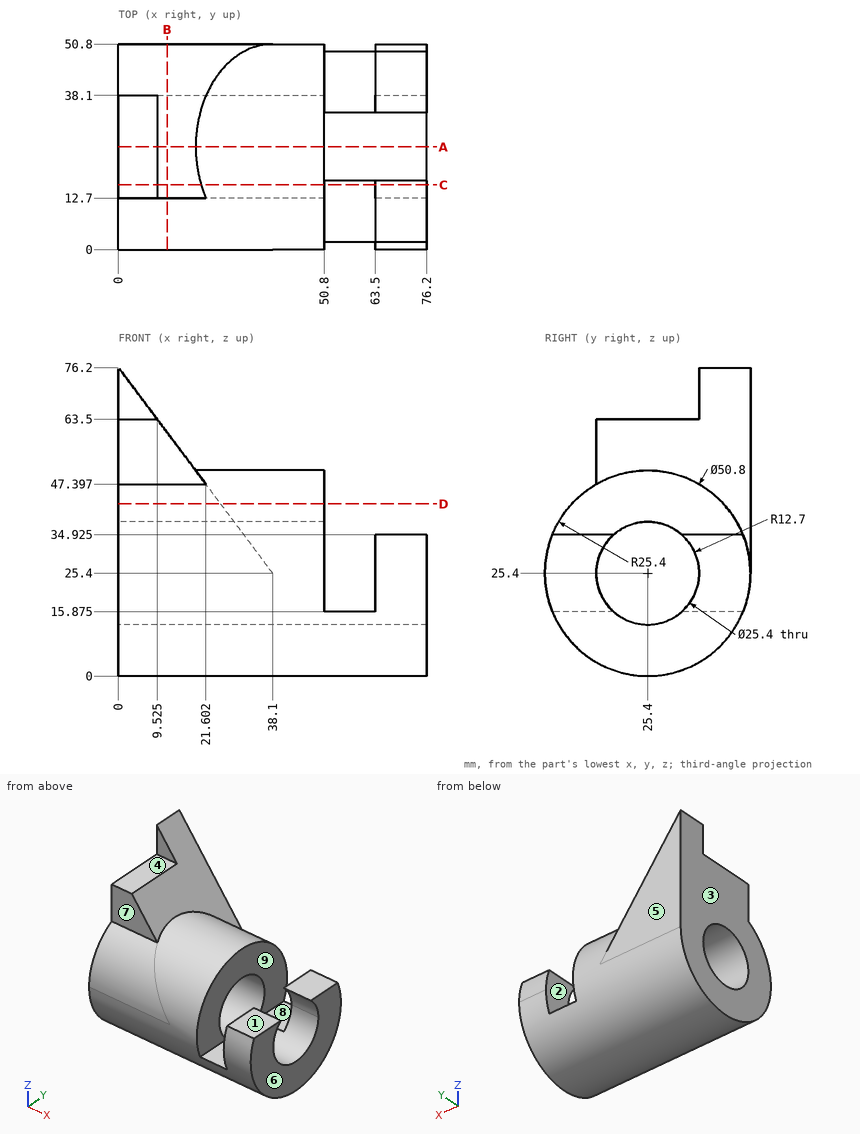
Answer from the drawing. Dimensions are ordinates in mm from the lowest x, y and z of the part. A direction names the side the tool comes from. Coordinates: 2 decimals unless noted, no trailing zeros. Order: outer loops, then holes, each group sorted by start corner. A loop starts at its lowest first (then second) coordinate and runs counter-clockwise, first axis right, second up. Notation, with made-up numbers: (-5.75, 55) - (6.25, 55) arc R21 ccw to (6.25, 82) - close; hole circle Ø2 at (11, 87.25). An arc over 180 degrees is marked (long way). Use one line per item in the form item = value.
(1) Section D-D, the plane z = 42.5 is taken. Give the vertices of the cut face in (x, y) (1 decimal).
Computed values:
outline = (0, 6.6) - (50.8, 6.6) - (50.8, 44.2) - (25.3, 44.2) - (25.3, 50.8) - (0, 50.8) - close
(2) For a pull along X with two mould halves and no side action, classify the marked faces 6, 7, 8 and 9 as pulls with the +X half, pulls with the -X half, needs draft (parallel to the pull), parting line crosses it, or undercut.
Computed values:
face_6 = pulls with the +X half
face_7 = needs draft
face_8 = undercut
face_9 = undercut
(3) Section C-C, the plane y = 16 is taken. Give the vertices of the cut face in (x, z) (1 decimal).
Computed values:
outline = (0, 1.8) - (76.2, 1.8) - (76.2, 16.9) - (63.5, 16.9) - (63.5, 15.9) - (50.8, 15.9) - (50.8, 16.9) - (0, 16.9) - close; (0, 33.9) - (50.8, 33.9) - (50.8, 49) - (20.4, 49) - (9.5, 63.5) - (0, 63.5) - close; (63.5, 33.9) - (76.2, 33.9) - (76.2, 34.9) - (63.5, 34.9) - close
(4) Which of the six approach directions +Z, -Z, +X, -X, +Y, -Y give full straight-line access (tool end or side, diameter ignored) to the marked faces 1, 2, 3, 4 and 5?
Computed values:
face_1 = +Z, +X, +Y, -Y
face_2 = +Z, +Y, -Y
face_3 = +Z, -Z, -X, +Y, -Y
face_4 = +Z, +X, -X, -Y
face_5 = +Z, -Z, +X, -X, +Y
(5) Straight lines are drawn through the part: L1, parallel to Y at x = 23, z = 25.4; L2, parallel to X at y = 36.5, z = 32. For each, find the intervals that lie inside material, in ascending order.
Computed values:
L1 = 0 to 12.7, 38.1 to 50.8
L2 = 0 to 50.8, 63.5 to 76.2
(6) Given pin 1 Ø6.5 at (x, y) = (60, 40.5) entering from +Z (3 decimals); pin 2 Ø5 at (x, z) = (7, 69) entering from -Y; pin 3 Ø5 at (x, y) = (7, 29) entering from +Z, each flat-ended and moving along its own axis, determine where each tip first touches the part or whether it passes through.
Computed values:
pin_1 = 15.875
pin_2 = 38.1
pin_3 = 63.5
(7) Section B-B, the plane x = 12 is taken. Give the vertices of the cut face in (y, z).
Computed values:
outline = (12.7, 47.4) arc R25.4 ccw (long way) to (50.8, 25.4) - (50.8, 60.2) - (12.7, 60.2) - close; hole circle Ø25.4 at (25.4, 25.4)
(8) Section A-A, the plane y = 25.4 is taken. Give the vertices of the cut face in (x, z) (3 decimals), then the cut area to 3 significant figures.
Computed values:
outline = (0, 0) - (76.2, 0) - (76.2, 12.7) - (0, 12.7) - close; (0, 38.1) - (50.8, 38.1) - (50.8, 50.8) - (19.05, 50.8) - (9.525, 63.5) - (0, 63.5) - close
area = 1,790 mm²
